Read the model definition and answer for the solid it produces. Units are mm, in the model's axes. Coordinates: 2 decimals unless noted, no trailing zeros. Write each loop counter-clockwise with the first axis right and the second up, starting at its lowest first coordinate (ties: lowest second). Pieces come first, ordered by that corner, then holes. Notation, with made-up numbers: (5, 34) -> (59, 34) arc R24 ccw to (59, 63) -> close; hole circle Ø11 at (79.25, 19.5). An arc over 180 degrees is marked (long way). Answer as a JSON object with one key per item and string values. Group by question number.
(1) Straight lines are drawn through the part: L1, parallel to Z at x = 3, y = 2.75; L2, parallel to Z at x = -2, y = 1.15; L3, parallel to X at y = 2.15, z = 33. For each, find the intervals that lie inside material, in ascending order.
(2) Find section A-A (y = 2.4). Give the vertices of the cut face in (x, z), then the cut area to 3 significant figures.
(3) Find section B-B (x = 14). Give the vertices of the cut face in (y, z), then the cut area to 3 significant figures.
(4) Find section C-C (x = 5). Give the vertices of the cut face in (y, z), then the cut area to 3 significant figures.
(5) Find section D-D (z = 1). Give the vertices of the cut face in (x, y), then the cut area to 3 significant figures.
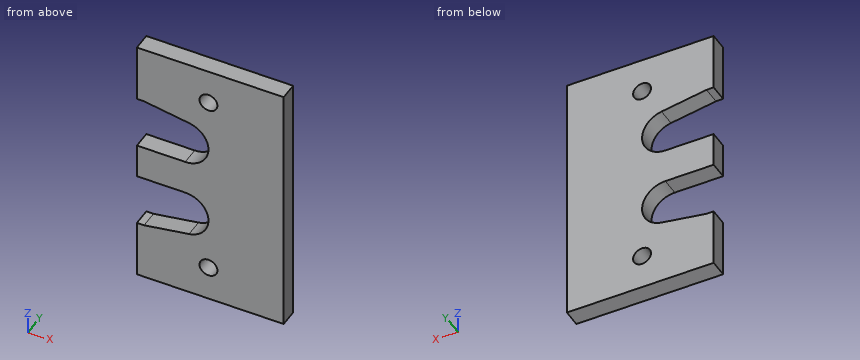
from build123d import *

# Parameters (mm, degrees)
SKETCH2_R           = 2.5
BOSS_EXTRUDE1_DEPTH = 5


with BuildPart() as part:
    # Sketch2 → Boss-Extrude1 (new body)
    with BuildSketch(Plane(origin=(0, 0, 0), x_dir=(1, 0, 0), z_dir=(0, 1, 0))):
        with BuildLine():
            Line((-5.298765278, -43.948074933), (35.701234722, -43.948074933))
            Line((35.701234722, -43.948074933), (35.701234722, 28.983136785))
            Line((35.701234722, 28.983136785), (-5.298765278, 28.983136785))
            Line((-5.298765278, 28.983136785), (-5.298765278, 12.448742644))
            Line((-5.298765278, 12.448742644), (-3.298765278, 12.448742644))
            Line((-3.298765278, 12.448742644), (9.26668749, 10.3608258))
            ThreePointArc((9.26668749, 10.3608258), (14.679218224, 3.414205702), (8.201234722, -2.551257356))
            Line((8.201234722, -2.551257356), (-5.298765278, -2.551257356))
            Line((-5.298765278, -2.551257356), (-5.298765278, -12.413680791))
            Line((-5.298765278, -12.413680791), (8.201234722, -12.413680791))
            ThreePointArc((8.201234722, -12.413680791), (14.679218224, -18.379143849), (9.26668749, -25.325763948))
            Line((9.26668749, -25.325763948), (-3.298765278, -27.413680791))
            Line((-3.298765278, -27.413680791), (-5.298765278, -27.413680791))
            Line((-5.298765278, -27.413680791), (-5.298765278, -43.948074933))
        make_face()
        with Locations(Location((14.701234722, -33.982469074, 0), (0, 0, 90))):
            Circle(SKETCH2_R, mode=Mode.SUBTRACT)
        with Locations(Location((14.701234722, 19.017530926, 0), (0, 0, 270))):
            Circle(SKETCH2_R, mode=Mode.SUBTRACT)
    extrude(amount=BOSS_EXTRUDE1_DEPTH)


solid = part.part
Results below:
{
 "1": {"L1": "z = -28.98 to -11.4, 2.55 to 12.41, 26.37 to 43.95", "L2": "z = -28.98 to -12.23, 2.55 to 12.41, 27.2 to 43.95", "L3": "x = -5.3 to 12.4, 17 to 35.7"},
 "2": {"outline": "(-5.3, -28.98) -> (35.7, -28.98) -> (35.7, 43.95) -> (-5.3, 43.95) -> (-5.3, 27.41) -> (-3.3, 27.41) -> (9.27, 25.33) arc R6.5 cw to (8.2, 12.41) -> (-5.3, 12.41) -> (-5.3, 2.55) -> (8.2, 2.55) arc R6.5 cw to (9.27, -10.36) -> (-3.3, -12.45) -> (-5.3, -12.45) -> close; hole circle Ø5 at (14.7, -19.02); hole circle Ø5 at (14.7, 33.98)", "area": "2,440 mm2"},
 "3": {"outline": "(0, -28.98) -> (5, -28.98) -> (5, -21.42) -> (0, -21.42) -> close; (0, -16.62) -> (5, -16.62) -> (5, -6.89) -> (0, -6.89) -> close; (0, -1.01) -> (5, -1.01) -> (5, 15.98) -> (0, 15.98) -> close; (0, 21.85) -> (5, 21.85) -> (5, 31.58) -> (0, 31.58) -> close; (0, 36.38) -> (5, 36.38) -> (5, 43.95) -> (0, 43.95) -> close", "area": "258 mm2"},
 "4": {"outline": "(0, -28.98) -> (5, -28.98) -> (5, -11.07) -> (0, -11.07) -> close; (0, 2.55) -> (5, 2.55) -> (5, 12.41) -> (0, 12.41) -> close; (0, 26.03) -> (5, 26.03) -> (5, 43.95) -> (0, 43.95) -> close", "area": "228 mm2"},
 "5": {"outline": "(12.42, 0) -> (35.7, 0) -> (35.7, 5) -> (12.42, 5) -> close", "area": "116 mm2"}
}
